Can you work these out from the model? Positions are in its coordinate system, mm. Give positions to 0.01 mm unless a question says otherwise; leave off trailing zeros. Order: outer loops, then holes, each group sorted by start corner. A loop starts at its lowest first (then second) coordinate and runs counter-clockwise, first axis right, second up. Notation, with made-up numbers: (34.5, -35) -> (59.5, -35) arc R28 cw to (59.5, -7) -> close; hole circle Ø7 at (-4.75, -31). An arc over 180 degrees is marked (long way). Answer as CSV lines item,"result".
```python
from build123d import *

# Parameters (mm, degrees)
SKETCH_1_W          = 245
SKETCH_1_H          = 120
SKETCH_1_R          = 15
EXTRUDE_1_DEPTH     = 2
FILLET_1_R          = 20
FILLET_2_R          = 20
SKETCH_3_R          = 1.6
CUT_EXTRUDE_1_DEPTH = 10


with BuildPart() as part:
    # 草图1 → 凸台-拉伸1 (new body)
    with BuildSketch(Plane.XY):
        with Locations((48.291102509, -15.293659776)):
            Rectangle(SKETCH_1_W, SKETCH_1_H)
        with Locations((-11.708897491, 14.706340224)):
            Circle(SKETCH_1_R, mode=Mode.SUBTRACT)
        with Locations((108.291102509, 14.706340224)):
            Circle(SKETCH_1_R, mode=Mode.SUBTRACT)
    extrude(amount=EXTRUDE_1_DEPTH)

    # 圆角1
    fillet_1_edges = [part.edges().sort_by_distance(p)[0] for p in [
        (170.791102509, -75.293659776, 1),
    ]]
    fillet(fillet_1_edges, radius=FILLET_1_R)

    # 圆角2
    fillet_2_edges = [part.edges().sort_by_distance(p)[0] for p in [
        (-74.208897491, -75.293659776, 1),
    ]]
    fillet(fillet_2_edges, radius=FILLET_2_R)

    # 草图3 → 切除-拉伸1 (cut)
    with BuildSketch(Plane.XY.offset(2)):
        with Locations((-26.208897491, -50.293659776)):
            Circle(SKETCH_3_R)
        with Locations((-57.208897491, -50.293659776)):
            Circle(SKETCH_3_R)
        with Locations((153.791102509, -50.293659776)):
            Circle(SKETCH_3_R)
        with Locations((122.791102509, -50.293659776)):
            Circle(SKETCH_3_R)
        with BuildLine():
            Line((-47.708897491, -59.293659776), (-47.708897491, -41.293659776))
            ThreePointArc((-47.708897491, -41.293659776), (-41.708897491, -35.293659776), (-35.708897491, -41.293659776))
            Line((-35.708897491, -41.293659776), (-35.708897491, -59.293659776))
            ThreePointArc((-35.708897491, -59.293659776), (-41.708897491, -65.293659776), (-47.708897491, -59.293659776))
        make_face()
        with BuildLine():
            Line((144.291102509, -59.293659776), (144.291102509, -41.293659776))
            ThreePointArc((144.291102509, -41.293659776), (138.291102509, -35.293659776), (132.291102509, -41.293659776))
            Line((132.291102509, -41.293659776), (132.291102509, -59.293659776))
            ThreePointArc((132.291102509, -59.293659776), (138.291102509, -65.293659776), (144.291102509, -59.293659776))
        make_face()
    extrude(amount=-CUT_EXTRUDE_1_DEPTH, mode=Mode.SUBTRACT)


solid = part.part
```
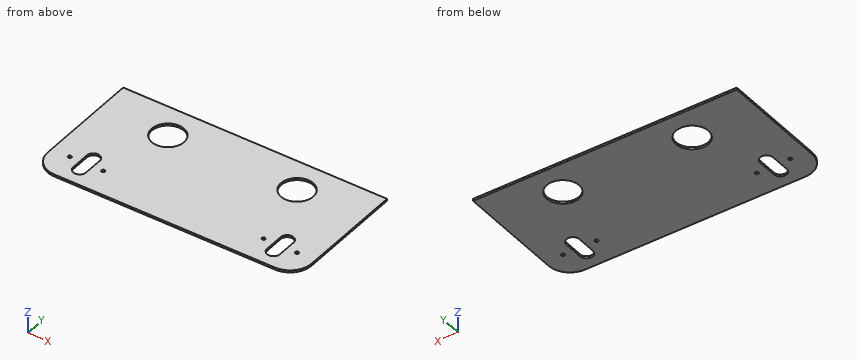
Item 1: For pin 1 (4 mm diameter, centred on x = 153.79, y = -50.29, fed in from +Z); pin 2 (2.5 mm diameter, centred on x = 122.79, y = -50.29, fed in from +Z), each with a flat end and sliding along its axis, tell me the tip position at first contact or that it passes through.
Numbers:
pin 1,"stops at z = 2"
pin 2,"passes through"
Item 2: Imagine slicing it at C-C, the plane z = 0.4. Give the number of separate pieces and of enclosed holes in the cut face, then the cut area to 3 significant figures.
Numbers:
separate pieces,"1"
enclosed holes,"8"
area,"27,100 mm²"
Item 3: Imagine slicing it at B-B, the plane x = 110. Please give me the cut outline in (y, z).
Numbers:
outline,"(-75.29, 0) -> (-0.2, 0) -> (-0.2, 2) -> (-75.29, 2) -> close; (29.61, 0) -> (44.71, 0) -> (44.71, 2) -> (29.61, 2) -> close"
Item 4: Imagine slicing it at D-D, the plane x = -40.5. Please give me the cut outline in (y, z), then the cut area to 3 significant figures.
Numbers:
outline,"(-75.29, 0) -> (-65.17, 0) -> (-65.17, 2) -> (-75.29, 2) -> close; (-35.42, 0) -> (44.71, 0) -> (44.71, 2) -> (-35.42, 2) -> close"
area,"180 mm²"
Item 5: Please list where these lines run through material, in increasing order: line 1 along X through (y, z) = (-46.5, 1.65); line 2 along X through (y, z) = (-38.5, 1.5); line 3 along Y through (x, z) = (-45, 1.8).
Numbers:
line 1,"x = -74.21 to -47.71, -35.71 to 132.29, 144.29 to 170.79"
line 2,"x = -74.21 to -47.02, -36.4 to 132.98, 143.6 to 170.79"
line 3,"y = -75.29 to -64.31, -36.28 to 44.71"
Item 6: Imagine slicing it at A-A, the plane y = -45.5. Please give me the cut outline in (x, z), then the cut area to 3 significant figures.
Numbers:
outline,"(-74.21, 0) -> (-47.71, 0) -> (-47.71, 2) -> (-74.21, 2) -> close; (-35.71, 0) -> (132.29, 0) -> (132.29, 2) -> (-35.71, 2) -> close; (144.29, 0) -> (170.79, 0) -> (170.79, 2) -> (144.29, 2) -> close"
area,"442 mm²"
